Source: CAD feature listing. Evaluate the final solid. Frame: model axes, mm. Face numbers are marked on the shaded views. Give positions to 0.01 mm unless a question says otherwise; leave off trailing zeros. Loops run counter-clockwise (first coordinate to the right, second up) from the corner with the lowest first, then second, coordinate; pieces in that order, holes last. Notation, with made-up numbers: M 46.5,88 L 59.5,88 A24 ccw 59.5,125 Z; hole C 77.5,29.25 d3. An arc over 180 degrees is marked long. Put each result on its own line as item: value.
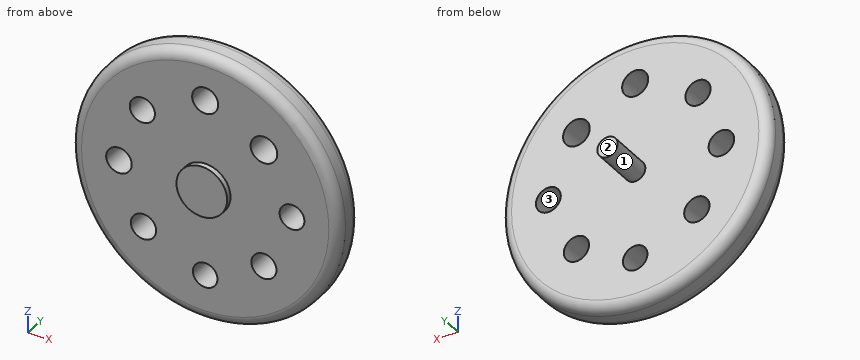
from build123d import *

# Parameters (mm, degrees)
F0_R     = 15.875
F1_DEPTH = 3.81
F3_R     = 1.454915
F3_R_2   = 1.498047
F3_R_3   = 1.514597
F3_R_4   = 1.491631
F3_R_5   = 1.471893
F3_R_6   = 1.580597
F3_R_7   = 1.544444
F4_DEPTH = 25.4
F6_R     = 1.22642
F7_R     = 1.202977
F8_DEPTH = 5.3594
F5_R     = 3.001673
F9_DEPTH = 0.6604


with BuildPart() as f1:
    # F0 (on Front) → F1 (new body)
    with BuildSketch(Plane.XZ):
        Circle(F0_R)
    extrude(amount=F1_DEPTH)

    # F3 (on face) → F4 (cut)
    with BuildSketch(Plane.XZ.offset(3.81)):
        with Locations((0, -10.367244)):
            Circle(F3_R)
        with Locations((-7.305188, -6.974129)):
            Circle(F3_R_2)
        with Locations((-10.213573, 0)):
            Circle(F3_R_3)
        with Locations((-7.443683, 6.944567)):
            Circle(F3_R_4)
        with Locations((10.28361, 0)):
            Circle(F3_R_5)
        with Locations((6.959744, -6.974129)):
            Circle(F3_R_4)
        with Locations((6.959744, 6.944567)):
            Circle(F3_R_6)
        with Locations((0, 10.545424)):
            Circle(F3_R_7)
    extrude(amount=-F4_DEPTH, mode=Mode.SUBTRACT)

    # F6
    f6_edges = [f1.edges().sort_by_distance(p)[0] for p in [
        (15.875, -1.905, 0),
        (-15.875, 0, 0),
        (-15.875, -3.81, 0),
    ]]
    fillet(f6_edges, radius=F6_R)

    # F7 (on face) → F8 (join)
    with BuildSketch(Plane(origin=(0, 0, 0), x_dir=(-1, 0, 0), z_dir=(0, 1, 0))):
        Circle(F7_R)
    extrude(amount=F8_DEPTH)

    # F5 (on face) → F9 (join)
    with BuildSketch(Plane.XZ.offset(3.81)):
        Circle(F5_R)
    extrude(amount=F9_DEPTH)


solid = f1.part
1. Section query B-B (x = 0). Output: boundary loops of the cut face in (y, z) (3 decimals).
Found:
outline: M -4.47,-3.002 L -3.81,-3.002 L -3.81,-8.912 L 0,-8.912 L 0,-1.203 L 5.359,-1.203 L 5.359,1.203 L 0,1.203 L 0,9.001 L -3.81,9.001 L -3.81,3.002 L -4.47,3.002 Z; M -3.81,-14.649 A1.226 ccw -2.584,-15.875 L -1.226,-15.875 A1.226 ccw 0,-14.649 L 0,-11.822 L -3.81,-11.822 Z; M -3.81,12.09 L 0,12.09 L 0,14.649 A1.226 ccw -1.226,15.875 L -2.584,15.875 A1.226 ccw -3.81,14.649 Z
2. Section query C-C (y = 3.25). Output: boundary loops of the cut face in (x, z).
Found:
outline: C 0,0 d2.41
3. Section query A-A (z = 0). Output: boundary loops of the cut face in (x, y) (1 decimal), plus the area to 3 significant figures.
Found:
outline: M -15.9,-2.6 A1.2 ccw -14.6,-3.8 L -11.7,-3.8 L -11.7,0 L -14.6,0 A1.2 ccw -15.9,-1.2 Z; M -8.7,-3.8 L -3,-3.8 L -3,-4.5 L 3,-4.5 L 3,-3.8 L 8.8,-3.8 L 8.8,0 L 1.2,0 L 1.2,5.4 L -1.2,5.4 L -1.2,0 L -8.7,0 Z; M 11.8,-3.8 L 14.6,-3.8 A1.2 ccw 15.9,-2.6 L 15.9,-1.2 A1.2 ccw 14.6,0 L 11.8,0 Z
area: 114 mm^2
4. Contact query for flat-ended pins moving along their axis: P1, Ø9, axis at x = -2.5, z = 6.5, coming from the +Y side; P2, Ø3, axis at y = -2.5, z = -4.5, coming from the -X side; P3, Ø2, axis at y = -3.5, z = -2, coming from the -X side. Output: stop coordinate, or through.
Found:
P1: y = 0
P2: x = -15.59
P3: x = -15.81
5. Material intervals for line 1 (Z direction, x = 0, y = -1.1); line 2 (X direction, y = -3, z = -7); line 3 (X direction, y = -2.5, z = -7.5), sorted ascending. Write a range as from..to.
Found:
line 1: -15.87..-11.82, -8.91..9, 12.09..15.87
line 2: -14.17..-8.8, -5.81..5.47, 8.45..14.17
line 3: -13.99..-8.71, -5.9..5.56, 8.36..13.99
6. Draft query along Z for the marked faces 1, 2 and 3. Return one class per face: pulls with the +Z half, pulls with the -Z half, needs draft (parallel to the pull), parting line crosses it, or undercut.
Found:
face 1: parting line crosses it
face 2: needs draft
face 3: undercut
7. Section query D-D (z = -6). State how many separate pieces and enclosed holes the cut face has, plus the area to 3 significant figures.
Found:
separate pieces: 3
enclosed holes: 0
area: 93.3 mm^2
